Part model, mm, in its own coordinate system. A direction names the side the tool comes from. Round coordinates to 2 decimals unless told otherwise and drop trailing zeros. Loops run counter-clockwise (first coordinate to the right, second up) from the corner with the lowest first, then second, coordinate; pieces in that order, holes last. Notation, with made-up numbers: (-24, -13.75) -> (26, -13.75) arc R21 ccw to (26, 23.25) -> close; hole circle Ø1 at (19, 39.25). An arc over 180 degrees is marked (long way). Answer as CSV lines item,"result".
from build123d import *

# Parameters (mm, degrees)
F0_R     = 2.1
F0_R_2   = 7.5
F0_R_3   = 5.25
F1_DEPTH = 4
F0_R_4   = 3.15
F2_DEPTH = 3.5


with BuildPart() as f1:
    # F0 (on Top) → F1 (new body)
    with BuildSketch(Plane.XY):
        with BuildLine():
            Line((30, -16), (30, 30))
            Line((30, 30), (-30, 30))
            Line((-30, 30), (-30, -30))
            Line((-30, -30), (16, -30))
            ThreePointArc((16, -30), (25.899495, -25.899495), (30, -16))
        make_face()
        with Locations((-20, -16)):
            Circle(F0_R, mode=Mode.SUBTRACT)
        with Locations((6, -16)):
            Circle(F0_R_2, mode=Mode.SUBTRACT)
        with Locations((-20, 4)):
            Circle(F0_R, mode=Mode.SUBTRACT)
        with Locations((-4, 20)):
            Circle(F0_R, mode=Mode.SUBTRACT)
        with Locations((6, 1.5)):
            Circle(F0_R_3, mode=Mode.SUBTRACT)
        with Locations((16, 20)):
            Circle(F0_R, mode=Mode.SUBTRACT)
    extrude(amount=-F1_DEPTH)

    # F0 (on Top) → F2 (join)
    with BuildSketch(Plane.XY):
        with Locations((6, -16)):
            Circle(F0_R_2)
        with Locations((6, -16)):
            Circle(F0_R_4, mode=Mode.SUBTRACT)
    extrude(amount=-F2_DEPTH)


solid = f1.part
Q1. Saw through at D-D, the plane y = 4. Write the cut outline in (x, z), then the cut area to 3 significant figures.
Geometry results:
outline,"(-30, -4) -> (-22.1, -4) -> (-22.1, 0) -> (-30, 0) -> close; (-17.9, -4) -> (1.38, -4) -> (1.38, 0) -> (-17.9, 0) -> close; (10.62, -4) -> (30, -4) -> (30, 0) -> (10.62, 0) -> close"
area,"186 mm2"
Q2. Saw through at C-C, the plane z = -1.85. Write the cut outline in (x, y), then the cut area to 3 significant figures.
Geometry results:
outline,"(-30, -30) -> (16, -30) arc R14 ccw to (30, -16) -> (30, 30) -> (-30, 30) -> close; hole circle Ø4.2 at (-20, -16); hole circle Ø4.2 at (-20, 4); hole circle Ø4.2 at (-4, 20); hole circle Ø10.5 at (6, 1.5); hole circle Ø6.3 at (6, -16); hole circle Ø4.2 at (16, 20)"
area,"3,380 mm2"
Q3. Saw through at A-A, the plane x = -4. Write the cut outline in (y, z).
Geometry results:
outline,"(-30, -4) -> (17.9, -4) -> (17.9, 0) -> (-30, 0) -> close; (22.1, -4) -> (30, -4) -> (30, 0) -> (22.1, 0) -> close"
Q4. Saw through at B-B, the plane x = -20. Write the cut outline in (y, z).
Geometry results:
outline,"(-30, -4) -> (-18.1, -4) -> (-18.1, 0) -> (-30, 0) -> close; (-13.9, -4) -> (1.9, -4) -> (1.9, 0) -> (-13.9, 0) -> close; (6.1, -4) -> (30, -4) -> (30, 0) -> (6.1, 0) -> close"
Q5. Two-plate mould, pull along Y, no slides. Class faces 1 (the face through (0, 0, 0)), 2 (the face through (-7, -30, -2)), 3 (the face through (17.13, 21.77, -1.97)): pulls with the +Y half, pulls with the -Y half, needs draft (parallel to the pull), parting line crosses it, or undercut.
Geometry results:
face 1,"needs draft"
face 2,"pulls with the -Y half"
face 3,"undercut"
Q6. Drill centre lines: line 1 along Y through (x, z) = (-20, -1.75); line 2 along Y through (x, z) = (6, -3.65); line 3 along X through (y, z) = (20.5, -0.95). Where is each one in solid material? Low to high.
Geometry results:
line 1,"-30 to -18.1, -13.9 to 1.9, 6.1 to 30"
line 2,"-30 to -23.5, -8.5 to -3.75, 6.75 to 30"
line 3,"-30 to -6.04, -1.96 to 13.96, 18.04 to 30"
Q7. Drop flat-ended pins along their axis: P1, Ø5, axis at x = -4, y = 20, coming from the +Z side; P2, Ø4, axis at x = -20, y = -16, coming from the +Z side; P3, Ø12, axis at x = 6, y = -16, coming from the -Z side. Give the stop position or say it passes through.
Geometry results:
P1,"z = 0"
P2,"through"
P3,"z = -3.5"
Q8. Which spindle directions (+Z, -Z, +X, -X, +Y, -Y) get a long thin tool onto all of the face, cutting with end or side? Do faces 4 (the face through (-17.997, -15.369, -1.972)), 5 (the face through (5.024, -8.564, -3.746)). Say none if no direction does.
Geometry results:
face 4,"+Z, -Z"
face 5,"-Z"
